Check sheet for the modelled part. Datum: model origin and axes. Units: mm. A direction names the side the tool comes from. Round coordinates to 2 decimals unless told otherwise and drop trailing zeros. Order: outer loops, then holes, each group sorted by start corner. A loop starts at its lowest first (then second) coordinate and runs counter-clockwise, first axis right, second up. Notation, with made-up numbers: M 3.25,40 L 42.25,40 A16 cw 42.25,53 Z; hole C 63,82 d11. An arc over 180 degrees is marked long. One line per item, written item: value. Start each with the question number.
(1) Cross-section at B-B, the plane y = 4.75. Enter the section's corners in (x, z) (3 decimals).
(2) Depth check by flat-ended pin: pin 1 Ø4 at (x, z) = (22, 1) entering from -Y; pin 2 Ø2 at (y, z) = (0.5, 7) entering from -X; pin 3 Ø3 at (y, z) = (-1, -0.5) entering from -X (3 decimals); pin 4 Ø3 at (x, y) = (9.5, 5) entering from -Z. Enter the tip coordinate at first touch or a pass-through.
(3) Release check for a two-part mould opening along X. For faces 4 (the face through (-13.08, -9.71, 0.03)), 5 (the face through (27.625, 0, 0)), 6 (the face through (16, -2, 3)), 7 (the face through (10.3, 0.2, -2)) record: released by +X, released by -X, zero draft, split by the parting line, or undercut.
(4) Cross-section at A-A, the plane x = -8.5. Enter the section's corners in (y, z).
(5) Thickness scan on L1, parallel to Y at x = -10, z = -0.5; L2, parallel to Z at x = 22, y = -8.75; L3, parallel to X at y = 1.5, z = 0.75 (3 decimals). Record the ranges inside material, lowest first.
(6) Access from +Z, -Z, +X, -X, +Y, -Y to the whole of each face (thin tool, end or side, straight path). Record for faces 1 (the face through (-2, 12.5, 0)), 2 (the face through (-13.17, 9.79, 0.03)), 3 (the face through (0, 9.5, 0)).
(7) Cross-section at C-C, the plane z = 1.25. Count the separate pieces of the cut face and the enclosed holes in it, and give its area (3 significant figures).
(8) Cross-section at D-D, the plane z = 8.25. Enter the section's corners in (x, y).
from build123d import *

# Parameters (mm, degrees)
F1_DEPTH = 2
F3_DEPTH = 2


with BuildPart() as f1:
    # F0 (on Top) → F1 (new body, symmetric)
    with BuildSketch(Plane.XY):
        Polygon((10.125, 9.5), (10.125, -9.5), (-10.125, -9.5), (-10.125, -7), (-16.125, -12.5), (-12.125, -12.5), (12.125, -12.5), (12.125, -2), (12.125, 0), (12.125, 2), (12.125, 12.5), (-12.125, 12.5), (-16.125, 12.5), (-10.125, 7), (-10.125, 9.5), align=None)
        with BuildLine():
            Line((17.0268920894, -5.8587268466), (12.125, -12.5))
            add(Edge.make_bspline(
                [(12.125, -12.5), (17.1111167669, -9.1784531251), (19.154572869, -9.144826131), (21.0990195423, -9.0642701834)],
                knots=[0, 0, 0, 0, 0.5479408527, 0.5479408527, 0.5479408527, 0.5479408527], degree=3))
            Line((21.0990195423, -9.0642701834), (17.0268920894, -5.8587268466))
        make_face()
        Polygon((12.125, -2), (12.125, -12.5), (17.0268920894, -5.8587268466), align=None)
        Polygon((12.125, 0), (12.125, -2), (19.875, -2), (27.625, -2), (27.625, 0), align=None)
        with BuildLine():
            Line((23.9668667925, -5.9598710895), (21.0990195423, -9.0642701834))
            add(Edge.make_bspline(
                [(21.0990195423, -9.0642701834), (22.7032162376, -8.9978103588), (24.2400222719, -8.8994083926), (27.625, -9.5)],
                knots=[0.5479408527, 0.5479408527, 0.5479408527, 0.5479408527, 1, 1, 1, 1], degree=3))
            Line((27.625, -9.5), (23.9668667925, -5.9598710895))
        make_face()
        Polygon((17.0268920894, -5.8587268466), (21.0990195423, -9.0642701834), (23.9668667925, -5.9598710895), (19.875, -2), align=None)
        Polygon((17.0268920894, 5.8587268466), (12.125, 12.5), (12.125, 2), align=None)
        with BuildLine():
            add(Edge.make_bspline(
                [(12.125, 12.5), (17.1111167669, 9.1784531251), (19.154572869, 9.144826131), (21.0990195423, 9.0642701834)],
                knots=[0, 0, 0, 0, 0.5479408527, 0.5479408527, 0.5479408527, 0.5479408527], degree=3))
            Line((12.125, 12.5), (17.0268920894, 5.8587268466))
            Line((17.0268920894, 5.8587268466), (21.0990195423, 9.0642701834))
        make_face()
        Polygon((12.125, 2), (12.125, 0), (27.625, 0), (27.625, 2), (19.875, 2), align=None)
        Polygon((27.625, -2), (19.875, -2), (23.9668667925, -5.9598710895), align=None)
        Polygon((23.9668667925, -5.9598710895), (27.625, -9.5), (27.625, -2), align=None)
        Polygon((23.9668667925, 5.9598710895), (21.0990195423, 9.0642701834), (17.0268920894, 5.8587268466), (19.875, 2), align=None)
        with BuildLine():
            add(Edge.make_bspline(
                [(21.0990195423, 9.0642701834), (22.7032162376, 8.9978103588), (24.2400222719, 8.8994083926), (27.625, 9.5)],
                knots=[0.5479408527, 0.5479408527, 0.5479408527, 0.5479408527, 1, 1, 1, 1], degree=3))
            Line((21.0990195423, 9.0642701834), (23.9668667925, 5.9598710895))
            Line((23.9668667925, 5.9598710895), (27.625, 9.5))
        make_face()
        Polygon((23.9668667925, 5.9598710895), (19.875, 2), (27.625, 2), align=None)
        Polygon((27.625, 2), (27.625, 9.5), (23.9668667925, 5.9598710895), align=None)
    extrude(amount=F1_DEPTH, both=True)

    # F2 (on Front) → F3 (join, symmetric)
    with BuildSketch(Plane.XZ):
        with BuildLine():
            Line((10.1918056607, 9.5617884584), (10.1918056607, 2.0617884584))
            Line((10.1918056607, 2.0617884584), (26.9152931869, 1.8099824665))
            ThreePointArc((26.9152931869, 1.8099824665), (18.2067231126, 4.9376539541), (10.1918056607, 9.5617884584))
        make_face()
    extrude(amount=F3_DEPTH, both=True)


solid = f1.part
Values found:
1. outline: M 10.125,-2 L 15.618,-2 L 15.618,2 L 10.125,2 Z; M 17.845,-2 L 27.625,-2 L 27.625,2 L 17.845,2 Z
2. pin 1: y = -9.12
2. pin 2: x = 10.19
2. pin 3: x = 10.125
2. pin 4: z = -2
3. face 4: released by -X
3. face 5: released by +X
3. face 6: undercut
3. face 7: zero draft
4. outline: M -12.5,-2 L -9.5,-2 L -9.5,2 L -12.5,2 Z; M 9.5,-2 L 12.5,-2 L 12.5,2 L 9.5,2 Z
5. L1: -12.5 to -9.5, 9.5 to 12.5
5. L2: -2 to 2
5. L3: 10.125 to 27.625
6. face 1: +Z, -Z, +X, -X, +Y
6. face 2: +Z, -Z, -X
6. face 3: +Z, -Z
7. separate pieces: 1
7. enclosed holes: 2
7. area: 478 mm^2
8. outline: M 10.19,-2 L 12.15,-2 L 12.15,2 L 10.19,2 Z
